Autodesk Inventor part; units mm, degrees
ref_plane "YZ Plane" through (0, 0, 0) normal (1, 0, 0) x (0, 1, 0)
ref_plane "XZ Plane" through (0, 0, 0) normal (0, 1, 0) x (-1, 0, 0)
ref_plane "XY Plane" through (0, 0, 0) normal (0, 0, 1) x (1, 0, 0)
sketch "Sketch1" plane through (0, 0, 0) normal (0, 1, 0) x (-1, 0, 0)
  line L0 (-25.2, 40) -> (-25.2, -40)
  line L1 (-25.2, -40) -> (25.2, -40)
  line L2 (25.2, -40) -> (25.2, 40)
  line L3 (25.2, 40) -> (-25.2, 40)
  line L4 (-25.2, 40) -> (25.2, -40) construction
  line L5 (-25.2, -40) -> (25.2, 40) construction
  point P0 (0, 0)
  dimension "d0" = 80
  dimension "d1" = 50.4
extrude "Extrusion1" add sketch "Sketch1" along normal blind 7.5
sketch "Sketch2" plane through (0, 7.5, 0) normal (0, 1, 0) x (1, 0, 0)
  line L0 (25.2, 40) -> (-25.2, 40)
  line L1 (-25.2, 40) -> (-15.2, 40)
  line L2 (-15.2, 40) -> (-15.2, -40)
  line L3 (-25.2, -40) -> (25.2, -40)
  line L4 (0, 40) -> (0, -40)
  line L5 (25.2, 40) -> (15.2, 40)
  line L6 (15.2, 40) -> (15.2, -40)
  line L7 (-14.2233, -40) -> (-14.2233, 40)
  line L8 (-14.2233, 40) -> (-16.1767, 40)
  line L9 (-16.1767, 40) -> (-16.1767, -40)
  line L10 (-16.1767, -40) -> (-14.2233, -40)
  line L11 (-14.2233, -40) -> (-16.1767, 40) construction
  line L12 (-14.2233, 40) -> (-16.1767, -40) construction
  point P0 (0, 0)
  point P1 (-15.2, 0)
  dimension "d4" = 10
  dimension "d5" = 10
sketch "Sketch3" plane through (-25.2, 0, 40) normal (0, 0, 1) x (1, 0, 0)
  point P0 (25.2, 0)
sketch "Sketch4" plane through (-25.2, 0, 40) normal (0, 0, 1) x (1, 0, 0)
  line L0 (0, 7.5) -> (50.4, 7.5)
  line L1 (9.0233, 7.5) -> (10.9782, 7.5)
  line L2 (9.0233, 7.5) -> (10.0298, 6.523)
  line L3 (10.0298, 6.523) -> (10.9782, 7.5)
  point P0 (25.2, 0)
extrude "Extrusion2" cut sketch "Sketch4" against normal up to surface (80 mm away)
ref_plane "Work Plane1" through (0, 0, -40) normal (-1, 0, 0) x (0, 0, 1)
mirror "Mirror1" about plane through (0, 0, -40) normal (-1, 0, 0) of "Extrusion2"
ref_plane "Work Plane2" through (12.6, 0, -40) normal (-1, 0, 0) x (0, 0, 1)
sketch "Sketch5" plane through (25.2, 0, -40) normal (0, 0, -1) x (-1, 0, 0)
  line L0 (39.4218, 7.5) -> (10.9782, 7.5)
  line L1 (25.2, 7.5) -> (24.2, 7.5)
  line L2 (24.2, 7.5) -> (24.2, 5.5)
  line L3 (24.2, 5.5) -> (26.2, 5.5)
  line L4 (26.2, 5.5) -> (26.2, 7.5)
  line L5 (24.2, 7.5) -> (26.2, 7.5)
  point P0 (25.2, 0)
  dimension "d8" = 1
  dimension "d9" = 2
  dimension "d10" = 2
extrude "Extrusion3" cut sketch "Sketch5" against normal up to surface (80 mm away)
ref_plane "Work Plane3" through (-25.2, 0, 0) normal (0, 0, 1) x (1, 0, 0)
properties part number "Circuit Board"
Design review of the part built by this model. Coordinates are the model's own, in mm. A direction names the side the tool comes from. Coordinates: 2 decimals unless noted, no trailing zeros. Order: outer loops, then holes, each group sorted by start corner. A loop starts at its lowest first (then second) coordinate and runs counter-clockwise, first axis right, second up. Notation, with made-up numbers: (-11, -8) - (9, -8) arc R29 cw to (9, 27) - close; hole circle Ø9 at (47.25, 17). An arc over 180 degrees is marked (long way). Put each result on its own line as item: value.
1) Wall thickness on L1, parallel to X at y = 5.75, z = -1.5; L2, parallel to Y at x = -0.5, z = -15.5: over which ranges is each line inside the solid? List them lowest first. Write a range as from..to.
Response values:
L1: x = -25.2..-1, 1..25.2
L2: y = 0..5.5
2) Take a section at A-A, the plane z = -6.5. Give the boundary of the cut face in (x, y).
Response values:
outline: (-25.2, 0) - (25.2, 0) - (25.2, 7.5) - (16.18, 7.5) - (15.17, 6.52) - (14.22, 7.5) - (1, 7.5) - (1, 5.5) - (-1, 5.5) - (-1, 7.5) - (-14.22, 7.5) - (-15.17, 6.52) - (-16.18, 7.5) - (-25.2, 7.5) - close
3) Insertion check: P1, Ø0.6, axis at x = 0, z = -20, coming from the +Y side. The pin has a flat end and moves straight along its axis. Give the tip position at first contact, or say it passes through.
Response values:
P1: stops at y = 5.5
4) Tool access review of faces 5 (the face through (-8, 7.5, 1)), 6 (the face through (1, 7, -1)): name each direction out of +Z, -Z, +X, -X, +Y, -Y from which nothing blocks a thin tool from reaching the whole face with its end or side.
Response values:
face 5: +Z, -Z, +X, -X, +Y
face 6: +Z, -Z, +Y
5) The part is to be moulded in two halves that separate along X. For faces 1 (the face through (0, 5.5, -1)), 2 (the face through (0, 4, 40)), 3 (the face through (-1, 6, -1)), 4 (the face through (-25.2, 4, -1)), say which applies: released by +X, released by -X, zero draft, split by the parting line, or undercut.
Response values:
face 1: undercut
face 2: zero draft
face 3: undercut
face 4: released by -X
6) Take a section at B-B, the plane x = 0. Give the boundary of the cut face in (y, z), and give its area (3 significant figures).
Response values:
outline: (0, -40) - (5.5, -40) - (5.5, 40) - (0, 40) - close
area: 440 mm²
